```python
from build123d import *

# Parameters (mm, degrees)
SKETCH1_W               = 76.2
SKETCH1_H               = 47.625
BOSS_EXTRUDE1_DEPTH     = 3.175
SKETCH2_W               = 76.2
SKETCH2_H               = 3.175
BOSS_EXTRUDE2_DEPTH     = 66.675
SKETCH6_W               = 12.7
SKETCH6_H               = 12.7
BOSS_EXTRUDE4_DEPTH     = 3.175
SKETCH7_W               = 12.7
SKETCH7_H               = 12.7
BOSS_EXTRUDE5_DEPTH     = 3.175
SKETCH8_W               = 12.7
SKETCH8_H               = 12.7
BOSS_EXTRUDE6_DEPTH     = 3.175
CUT_EXTRUDE4_DEPTH      = 3.175
CUT_EXTRUDE5_DEPTH      = 1
CUT_EXTRUDE5_DEPTH_BACK = 77.2
SKETCH11_R              = 3.175
CUT_EXTRUDE6_DEPTH      = 3.175
CUT_EXTRUDE7_DEPTH      = 3.175


with BuildPart() as part:
    # Sketch1 → Boss-Extrude1 (new body)
    with BuildSketch(Plane.XY):
        Rectangle(SKETCH1_W, SKETCH1_H)
    extrude(amount=BOSS_EXTRUDE1_DEPTH)

    # Sketch2 → Boss-Extrude2 (add)
    with BuildSketch(Plane(origin=(0, 0, 0), x_dir=(-1, 0, 0), z_dir=(0, 0, -1))):
        with Locations((0, -19.05)):
            Rectangle(SKETCH2_W, SKETCH2_H)
    extrude(amount=BOSS_EXTRUDE2_DEPTH)

    # Sketch6 → Boss-Extrude4 (add)
    with BuildSketch(Plane(origin=(38.1, 0, 0), x_dir=(0, 0, -1), z_dir=(1, 0, 0))):
        with Locations((6.35, 14.2875)):
            Rectangle(SKETCH6_W, SKETCH6_H)
    extrude(amount=-BOSS_EXTRUDE4_DEPTH)

    # Sketch7 → Boss-Extrude5 (add)
    with BuildSketch(Plane.ZY.offset(38.1)):
        with Locations((-6.35, 14.2875)):
            Rectangle(SKETCH7_W, SKETCH7_H)
    extrude(amount=-BOSS_EXTRUDE5_DEPTH)

    # Sketch8 → Boss-Extrude6 (add)
    with BuildSketch(Plane(origin=(0, 0, -66.675), x_dir=(-1, 0, 0), z_dir=(0, 0, -1))):
        with Locations((0, -11.1125)):
            Rectangle(SKETCH8_W, SKETCH8_H)
    extrude(amount=-BOSS_EXTRUDE6_DEPTH)

    # Sketch9 → Cut-Extrude4 (cut)
    with BuildSketch(Plane(origin=(0, 0, -66.675), x_dir=(-1, 0, 0), z_dir=(0, 0, -1))):
        Polygon((2.522327856, -6.7437), (-2.522327856, -6.7437), (-5.044655712, -11.1125), (-2.522327856, -15.4813), (2.522327856, -15.4813), (5.044655712, -11.1125), align=None)
    extrude(amount=-CUT_EXTRUDE4_DEPTH, mode=Mode.SUBTRACT)

    # Sketch10 → Cut-Extrude5 (cut, two sides)
    with BuildSketch(Plane(origin=(38.1, 0, 0), x_dir=(0, 0, -1), z_dir=(1, 0, 0))) as cut_extrude5_sk:
        Polygon((10.7188, 11.765172144), (10.7188, 16.809827856), (6.35, 19.332155712), (1.9812, 16.809827856), (1.9812, 11.765172144), (6.35, 9.242844288), align=None)
    extrude(amount=CUT_EXTRUDE5_DEPTH, mode=Mode.SUBTRACT)
    extrude(cut_extrude5_sk.sketch, amount=-CUT_EXTRUDE5_DEPTH_BACK, mode=Mode.SUBTRACT)

    # Sketch11 → Cut-Extrude6 (cut)
    with BuildSketch(Plane.XY.offset(3.175)):
        with Locations((-25.4, 14.2875)):
            Circle(SKETCH11_R)
    extrude(amount=-CUT_EXTRUDE6_DEPTH, mode=Mode.SUBTRACT)

    # Sketch12 → Cut-Extrude7 (cut)
    with BuildSketch(Plane(origin=(0, -17.4625, 0), x_dir=(1, 0, 0), z_dir=(0, 1, 0))):
        Polygon((-8.983187105, 5.5499), (-8.066643552, 3.9624), (-6.233556448, 3.9624), (-5.317012895, 5.5499), (-6.233556448, 7.1374), (-8.066643552, 7.1374), align=None)
        Polygon((32.831643552, 3.6322), (33.748187105, 5.2197), (32.831643552, 6.8072), (30.998556448, 6.8072), (30.082012895, 5.2197), (30.998556448, 3.6322), align=None)
        Polygon((33.748187105, 58.2549), (32.831643552, 59.8424), (30.998556448, 59.8424), (30.082012895, 58.2549), (30.998556448, 56.6674), (32.831643552, 56.6674), align=None)
        Polygon((-30.998556448, 29.3624), (-32.831643552, 29.3624), (-33.748187105, 27.7749), (-32.831643552, 26.1874), (-30.998556448, 26.1874), (-30.082012895, 27.7749), align=None)
        Polygon((-30.082012895, 58.2549), (-30.998556448, 59.8424), (-32.831643552, 59.8424), (-33.748187105, 58.2549), (-32.831643552, 56.6674), (-30.998556448, 56.6674), align=None)
    extrude(amount=-CUT_EXTRUDE7_DEPTH, mode=Mode.SUBTRACT)


solid = part.part
```
Geometry check sheet. Reference: the model listing, model coordinates, mm. A direction names the side the tool comes from. Coordinates: 2 decimals unless noted, no trailing zeros. Loops run counter-clockwise (first coordinate to the right, second up) from the corner with the lowest first, then second, coordinate; pieces in that order, holes last. Notation, with made-up numbers: (24.25, 19.5) -> (31.25, 19.5) arc R26 ccw to (31.25, 35.5) -> close; hole circle Ø6 at (51.5, 41). An arc over 180 degrees is marked (long way). Put each result on its own line as item: value.
1) Thickness scan on line 1 (X direction, y = 14, z = -1) (3 decimals); line 2 (Y direction, x = -25.4, z = 1.35); line 3 (Y direction, x = -23, z = -49). Record the ranges inside material, lowest first.
Result set:
line 1: x = -38.1 to -34.925, 34.925 to 38.1
line 2: y = -23.81 to 11.11, 17.46 to 23.81
line 3: y = -20.64 to -17.46
2) Gauge pin test, flat ends, axial feed: pin 1 Ø1.6 at (x, y) = (36, 15) entering from -Z; pin 2 Ø2 at (x, z) = (25.5, -56) entering from -Y; pin 3 Ø2.5 at (x, z) = (36.5, -4) entering from +Y. Record the tip position at first contact, or that the pin passes through.
Result set:
pin 1: stops at z = -12.7
pin 2: stops at y = -20.64
pin 3: stops at y = 20.64
3) Cross-section at C-C on x = -25.4. Record the boundary of the cut face in (y, z) (1 decimal), plus the area to 3 significant figures.
Result set:
outline: (-23.8, 0) -> (-20.6, 0) -> (-20.6, -66.7) -> (-17.5, -66.7) -> (-17.5, 0) -> (11.1, 0) -> (11.1, 3.2) -> (-23.8, 3.2) -> close; (17.5, 0) -> (23.8, 0) -> (23.8, 3.2) -> (17.5, 3.2) -> close
area: 343 mm^2
4) Cross-section at A-A on x = -0.5. Record the boundary of the cut face in (y, z) (1 decimal).
Result set:
outline: (-23.8, 0) -> (-20.6, 0) -> (-20.6, -66.7) -> (-15.5, -66.7) -> (-15.5, -63.5) -> (-17.5, -63.5) -> (-17.5, 0) -> (23.8, 0) -> (23.8, 3.2) -> (-23.8, 3.2) -> close; (-6.7, -66.7) -> (-4.8, -66.7) -> (-4.8, -63.5) -> (-6.7, -63.5) -> close
5) Release check for a two-part mould opening along X. For faces 1 (the flat face through (-36.49, 10.486, -8.504)), 2 (the flat face through (-7, -19, -7.137)), 3 (the flat face through (6.35, -11, -65)) record: released by +X, released by -X, zero draft, split by the parting line, or undercut.
Result set:
face 1: zero draft
face 2: undercut
face 3: released by +X
6) Tool access check on faces 4 (the flat face through (0, -6.744, -65)), 5 (the flat face through (-36, 14, -10.719)), 6 (the flat face through (-1, 0, 3.175)), 7 (the flat face through (-32, -19, -56.667)), 8 (the flat face through (37, 14, -12.7)). Record the directions out of +Z, -Z, +X, -X, +Y, -Y that give a thin tool (end or side, any length) a straight path to the whole face; none if there is none.
Result set:
face 4: -Z
face 5: +X, -X
face 6: +Z, +X, -X, +Y, -Y
face 7: +Y, -Y
face 8: -Z, +X, -X, +Y
7) Cross-section at D-D on y = 5.5. Record the boundary of the cut face in (x, z) (3 decimals), plus the area to 3 significant figures.
Result set:
outline: (-38.1, 0) -> (38.1, 0) -> (38.1, 3.175) -> (-38.1, 3.175) -> close
area: 242 mm^2
8) Cross-section at B-B on x = 20.5. Record the boundary of the cut face in (y, z) (1 decimal), plus the area to 3 significant figures.
Result set:
outline: (-23.8, 0) -> (-20.6, 0) -> (-20.6, -66.7) -> (-17.5, -66.7) -> (-17.5, 0) -> (23.8, 0) -> (23.8, 3.2) -> (-23.8, 3.2) -> close
area: 363 mm^2
